from build123d import *

# Parameters (mm, degrees)
F1_DEPTH = 3.175
F3_DEPTH = 1.27
F4_R     = 3.175
F5_DEPTH = 25.4


with BuildPart() as f1:
    # F0 (on Top) → F1 (new body)
    with BuildSketch(Plane.XY):
        Polygon((0, 76.2), (0, 0), (76.2, 0), (76.2, 25.4), (25.4, 25.4), (25.4, 76.2), align=None)
    extrude(amount=F1_DEPTH)

    # F2 (on face) → F3 (cut)
    with BuildSketch(Plane.XY.offset(3.175)):
        Polygon((25.4, 25.4), (25.4, 76.2), (22.225, 76.2), (22.225, 25.4), (22.225, 22.225), (25.4, 22.225), (76.2, 22.225), (76.2, 25.4), align=None)
    extrude(amount=-F3_DEPTH, mode=Mode.SUBTRACT)

    # F4 (on face) → F5 (cut)
    with BuildSketch(Plane.XY.offset(3.175)):
        with Locations((69.85, 15.875)):
            Circle(F4_R)
        with Locations((57.15, 15.875)):
            Circle(F4_R)
        with Locations((15.875, 69.85)):
            Circle(F4_R)
        with Locations((15.875, 57.15)):
            Circle(F4_R)
    extrude(amount=-F5_DEPTH, mode=Mode.SUBTRACT)


solid = f1.part
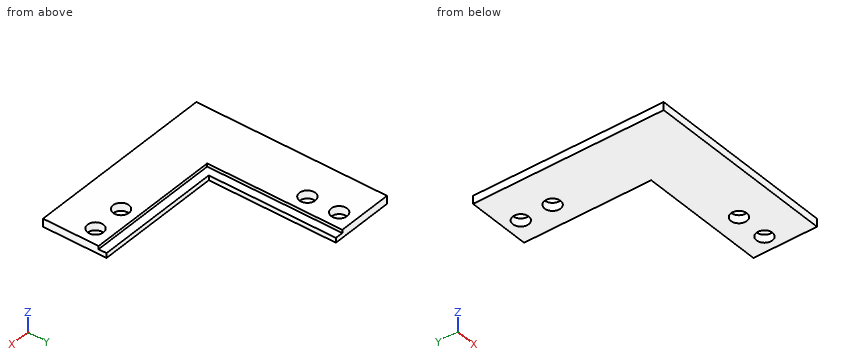
Here's how the part is built. I have some questions about the finished solid (model axes, mm). Round coordinates to 2 decimals unless told otherwise and drop trailing zeros. Write each loop counter-clockwise with the first axis right and the second up, starting at its lowest first coordinate (ties: lowest second). Pieces come first, ordered by that corner, then holes.
1. Suppose I cut it at A-A (x = 69.85). List the corners of the cut face in (y, z) for me (3 decimals).
2. Will these pins go through, and if not, where does the flat tip stop? pin 1 Ø1 at (x, z) = (62.5, 1) entering from +Y; pin 2 Ø0.6 at (y, z) = (52.5, 0.5) entering from +X.
3. I need wall thicknesses on L1, parallel to Y at x = 57.5, z = 1.3; L2, parallel to X at y = 13, z = 1.7; L3, parallel to X at y = 50, z = 1.2. Which ranges of each line are inside material? Lowest first, please.
4. Suppose I cut it at C-C (z = 0.95). List the corners of the cut face in (x, y) for me (3 decimals).
Answer sheet:
1. outline: (0, 0) - (12.7, 0) - (12.7, 3.175) - (0, 3.175) - close; (19.05, 0) - (25.4, 0) - (25.4, 1.905) - (22.225, 1.905) - (22.225, 3.175) - (19.05, 3.175) - close
2. pin 1: stops at y = 25.4
2. pin 2: stops at x = 25.4
3. L1: y = 0 to 12.72, 19.03 to 25.4
3. L2: x = 0 to 55.8, 58.5 to 68.5, 71.2 to 76.2
3. L3: x = 0 to 25.4
4. outline: (0, 0) - (76.2, 0) - (76.2, 25.4) - (25.4, 25.4) - (25.4, 76.2) - (0, 76.2) - close; hole circle Ø6.35 at (15.875, 57.15); hole circle Ø6.35 at (15.875, 69.85); hole circle Ø6.35 at (57.15, 15.875); hole circle Ø6.35 at (69.85, 15.875)
